from build123d import *

# Parameters (mm, degrees)
SKETCH1_R           = 22.5
BOSS_EXTRUDE1_DEPTH = 60
SKETCH2_R           = 14.25
CUT_EXTRUDE1_DEPTH  = 20


with BuildPart() as part:
    # Sketch1 → Boss-Extrude1 (new body)
    with BuildSketch(Plane(origin=(0, 0, 0), x_dir=(1, 0, 0), z_dir=(0, 1, 0))):
        with Locations(Location((0, 0, 0), (0, 0, 270))):
            Circle(SKETCH1_R)
        with BuildLine():
            Line((1.767766953, 1.767766953), (-1.767766953, 1.767766953))
            ThreePointArc((-1.767766953, 1.767766953), (0, -2.5), (1.767766953, 1.767766953))
        make_face(mode=Mode.SUBTRACT)
    extrude(amount=BOSS_EXTRUDE1_DEPTH)

    # Sketch2 → Cut-Extrude1 (cut)
    with BuildSketch(Plane(origin=(0, 60, 0), x_dir=(1, 0, 0), z_dir=(0, 1, 0))):
        with Locations(Location((0, 0, 0), (0, 0, 270))):
            Circle(SKETCH2_R)
    extrude(amount=-CUT_EXTRUDE1_DEPTH, mode=Mode.SUBTRACT)

    # Sketch4 → Cut-Revolve3 (revolve, cut)
    with BuildSketch(Plane.XY, mode=Mode.PRIVATE) as cut_revolve3_sk:
        Polygon((22.5, 5), (22.5, 55), (15, 47.5), (15, 12.5), align=None)
    revolve(cut_revolve3_sk.sketch.rotate(Axis((0, -24.387590134, 0), (0, 1, 0)), 90), axis=Axis((0, -24.387590134, 0), (0, 1, 0)), mode=Mode.SUBTRACT)


solid = part.part
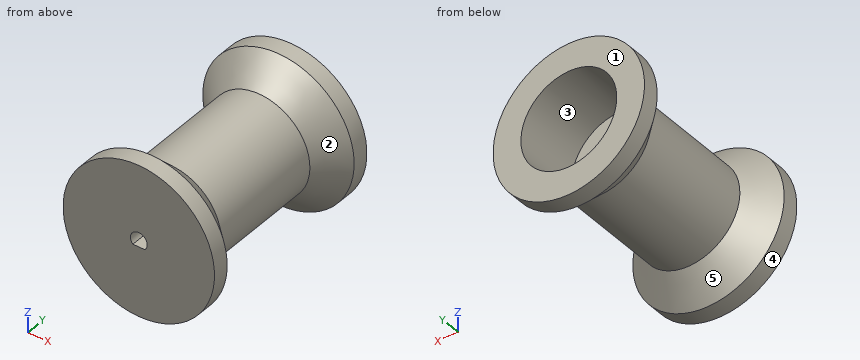
Here's how the part is built. I have some questions about the finished solid (model axes, mm). Face numbers are marked on the shaded views. A direction names the side the tool comes from. Give positions to 0.01 mm unless a question says otherwise; leave off trailing zeros. Order: outer loops, then holes, each group sorted by start corner. A loop starts at its lowest first (then second) coordinate and runs counter-clockwise, first axis right, second up. Notation, with made-up numbers: (17, -13.5) -> (33, -13.5) arc R6 cw to (33, -2.5) -> close; hole circle Ø10 at (-17, 25). An arc over 180 degrees is marked (long way). One line per item, written item: value. Start each with the question number.
1. Imagine slicing it at B-B, the plane x = 0. List the corners of the cut face in (y, z) for me, plus the area to 3 significant figures.
2. For the marked faces 4 and 5, which set-ups out of +Z, -Z, +X, -X, +Y, -Y let a thin tool reach every point of the face, with its end or its side?
3. Will these pins go through, and if not, where does the flat tip stop? pin 1 Ø14 at (x, z) = (4.5, 0) entering from +Y; pin 2 Ø12 at (x, y) = (10, 32) entering from +Z; pin 3 Ø5 at (y, z) = (46.5, -18) entering from +X; pin 4 Ø10 at (x, y) = (-9, 46.5) entering from +Z.
4. We'd pull the mould along Z, two halves only. Please class the marked faces 1, 2 and 3: released by +Z, released by -Z, zero draft, split by the parting line, or undercut.
5. I need wall thicknesses on probe 1 along X at (y, z) = (14, 0); probe 2 along X at (y, z) = (47.5, 0); probe 3 along Y at (x, z) = (10, -7). Which ranges of each line are inside material? Lowest first, please. Write a range as from..to.
6. Imagine slicing it at D-D, the plane y = 11. List the corners of the cut face in (x, z) for me, plus the area to 3 significant figures.
7. Imagine slicing it at A-A, the plane z = 0. List the corners of the cut face in (x, y) for me.
8. Imagine slicing it at C-C, the plane y = 25.5. List the corners of the cut face in (x, z) for me, plus the area to 3 significant figures.
Values follow:
1. outline: (0, -22.5) -> (5, -22.5) -> (12.5, -15) -> (47.5, -15) -> (55, -22.5) -> (60, -22.5) -> (60, -14.25) -> (40, -14.25) -> (40, -1.77) -> (0, -1.77) -> close; (0, 2.5) -> (40, 2.5) -> (40, 14.25) -> (60, 14.25) -> (60, 22.5) -> (55, 22.5) -> (47.5, 15) -> (12.5, 15) -> (5, 22.5) -> (0, 22.5) -> close
1. area: 1,320 mm2
2. face 4: +Y, -Y
2. face 5: none
3. pin 1: stops at y = 40
3. pin 2: stops at z = 14.46
3. pin 3: passes through
3. pin 4: stops at z = 17.22
4. face 1: zero draft
4. face 2: split by the parting line
4. face 3: undercut
5. probe 1: x = -15..-2.5, 2.5..15
5. probe 2: x = -15..-14.25, 14.25..15
5. probe 3: y = 0..40
6. outline: circle Ø33 at (0, 0); hole (-1.77, -1.77) -> (1.77, -1.77) arc R2.5 ccw (long way) to start
6. area: 837 mm2
7. outline: (-22.5, 0) -> (-2.5, 0) -> (-2.5, 40) -> (-14.25, 40) -> (-14.25, 60) -> (-22.5, 60) -> (-22.5, 55) -> (-15, 47.5) -> (-15, 12.5) -> (-22.5, 5) -> close; (2.5, 0) -> (22.5, 0) -> (22.5, 5) -> (15, 12.5) -> (15, 47.5) -> (22.5, 55) -> (22.5, 60) -> (14.25, 60) -> (14.25, 40) -> (2.5, 40) -> close
8. outline: circle Ø30 at (0, 0); hole (-1.77, -1.77) -> (1.77, -1.77) arc R2.5 ccw (long way) to start
8. area: 689 mm2
